Geometry check sheet. Reference: the model listing, model coordinates, mm. Face numbers are marked on the shaded views. A direction names the side the tool comes from. Give positions to 0.01 mm unless a question says otherwise; leave off trailing zeros. Order: outer loops, then holes, each group sorted by start corner. A loop starts at its lowest first (then second) coordinate and runs counter-clockwise, first axis right, second up. Notation, with made-up numbers: M 69,73.25 L 104,73.25 A4 cw 104,80.25 Z; hole C -13.75,76.25 d4. An arc over 180 degrees is marked long. Answer as CSV lines item,"result". Start each with the question number.
Q1. Thickness scan on line 1 (Z direction, x = 0, y = 31.5); line 2 (X direction, y = 9.5, z = 11); line 3 (Y direction, x = -1.5, z = -3.25). Record the ranges inside material, lowest first.
Q2. Go/stop test with a flat-tipped pin: pin 1 (4 mm diameter, centred on x = 3.5, z = 14, fed in from -Y). Record where the tip stops, or that it passes through.
Q3. Section check A-A, the plane z = 2.5. Record the boundary of the cut face in (x, y).
Q4. Section check C-C, the plane y = 19. Record the boundary of the cut face in (x, z), then the cut area to 3 significant figures.
Q5. Set-up check for the marked faces 1 and 2: record each of +Z, -Z, +X, -X, +Y, -Y from which the full face is reachable in a straight line by a thin tool's end or side.
Q6. Section check B-B, the plane x = 3.75. Record the boundary of the cut face in (y, z).
Q7. Section check D-D, the plane x = -6.25. Record the boundary of the cut face in (y, z), then the cut area to 3 significant figures.
Q8. Mould release check, pull along Z, two halves, no side actions. Record for the marked faces 3, 4 and 5: +Z half, -Z half, draft (parallel to the pull), parting line (faces both ways), or undercut.
Autodesk Inventor part; units mm, degrees
ref_plane "YZ Plane" through (0, 0, 0) normal (1, 0, 0) x (0, 1, 0)
ref_plane "XZ Plane" through (0, 0, 0) normal (0, 1, 0) x (-1, 0, 0)
ref_plane "XY Plane" through (0, 0, 0) normal (0, 0, 1) x (1, 0, 0)
sketch "Sketch1" plane through (0, 0, 0) normal (0, 1, 0) x (-1, 0, 0)
  line L0 (-6.7886, -4.7076) -> (18.6114, -4.7076)
  line L1 (18.6114, -4.7076) -> (18.6114, 20.6924)
  line L2 (18.6114, 20.6924) -> (-6.7886, 20.6924)
  line L3 (-6.7886, 20.6924) -> (-6.7886, -4.7076)
  line L4 (-5.2011, -3.1201) -> (17.0239, -3.1201)
  line L5 (17.0239, -3.1201) -> (17.0239, 19.1049)
  line L6 (17.0239, 19.1049) -> (-5.2011, 19.1049)
  line L7 (-5.2011, 19.1049) -> (-5.2011, -3.1201)
  point P0 (0, 0)
  dimension "d0" = 25.4
  dimension "d1" = 25.4
  dimension "d2" = 1.5875
  dimension "d3" = 1.5875
  dimension "d4" = 1.5875
  dimension "d5" = 1.5875
extrude "Extrusion1" add sketch "Sketch1" along normal blind 101.6
sketch "Sketch2" plane through (-18.6114, 0, 20.6924) normal (0, 0, 1) x (1, 0, 0)
  circle A0 centre (12.7, 8.255) radius 6.35
  circle A1 centre (12.7, 93.345) radius 6.35
  point P0 (25.4, 0)
  point P1 (25.4, 101.6)
  point P2 (18.6114, 0)
  dimension "d8" = 12.7
  dimension "d9" = 12.7
  dimension "d10" = 8.255
  dimension "d11" = 8.255
extrude "Extrusion2" cut sketch "Sketch2" against normal blind 101.6
fillet "Fillet1" radius 6.35 1 edges at (6.7886, 101.6, 7.9924)
fillet "Fillet2" radius 6.35 3 edges at (-18.6114, 101.6, 7.9924) (6.7886, 0, 7.9924) (-18.6114, 0, 7.9924)
equation "\"d3\" = d2"
equation "\"d4\" = d2"
equation "\"d5\" = d2"
properties part number "4inLink"
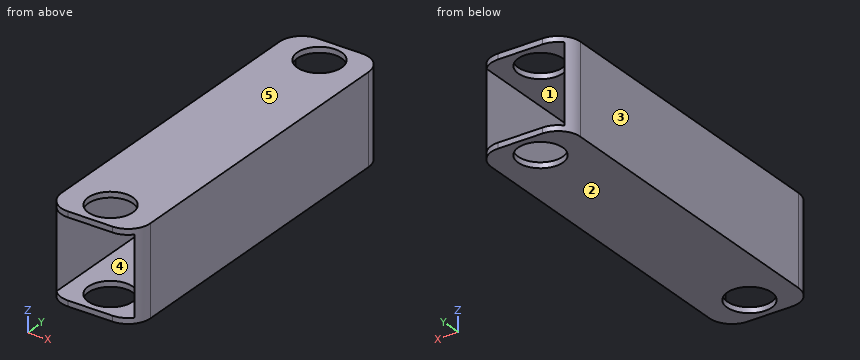
Answer block:
1,line 1,"z = -4.71 to -3.12, 19.1 to 20.69"
1,line 2,"x = -18.61 to -17.02, 5.2 to 6.79"
1,line 3,"y = 0 to 3.69, 12.82 to 88.78, 97.91 to 101.6"
2,pin 1,"stops at y = 2.15"
3,outline,"M -18.61,6.35 A6.35 ccw -17.02,2.15 L -17.02,99.45 A6.35 ccw -18.61,95.25 Z; M 5.2,2.15 A6.35 ccw 6.79,6.35 L 6.79,95.25 A6.35 ccw 5.2,99.45 Z"
4,outline,"M -18.61,-4.71 L 6.79,-4.71 L 6.79,20.69 L -18.61,20.69 Z; hole M -17.02,-3.12 L 5.2,-3.12 L 5.2,19.1 L -17.02,19.1 Z"
4,area,"151 mm2"
5,face 1,"+Y, -Y"
5,face 2,"-Z, +X, -X, +Y, -Y"
6,outline,"M 0.93,-4.71 L 100.67,-4.71 L 100.67,-3.12 L 0.93,-3.12 Z; M 0.93,19.1 L 100.67,19.1 L 100.67,20.69 L 0.93,20.69 Z"
7,outline,"M 0,-4.71 L 1.91,-4.71 L 1.91,-3.12 L 0,-3.12 Z; M 0,19.1 L 1.91,19.1 L 1.91,20.69 L 0,20.69 Z; M 14.6,-4.71 L 87,-4.71 L 87,-3.12 L 14.6,-3.12 Z; M 14.6,19.1 L 87,19.1 L 87,20.69 L 14.6,20.69 Z; M 99.69,-4.71 L 101.6,-4.71 L 101.6,-3.12 L 99.69,-3.12 Z; M 99.69,19.1 L 101.6,19.1 L 101.6,20.69 L 99.69,20.69 Z"
7,area,"242 mm2"
8,face 3,"draft"
8,face 4,"undercut"
8,face 5,"+Z half"
